from build123d import *

# Parameters (mm, degrees)
BOSS_EXTRUDE1_DEPTH = 1.5
SKETCH2_W           = 1.5
SKETCH2_H           = 5.2
SKETCH2_W_2         = 21.5
SKETCH2_H_2         = 1.5
BOSS_EXTRUDE2_DEPTH = 15


with BuildPart() as part:
    # Sketch1 → Boss-Extrude1 (new body)
    with BuildSketch(Plane.XY):
        Polygon((0, 0), (81.5, 0), (81.5, 13), (79, 13), (79, 10), (76.5, 10), (76.5, 5), (5, 5), (5, 10), (2.5, 10), (2.5, 20.5), (5, 20.5), (5, 25.5), (76.5, 25.5), (76.5, 20.5), (79, 20.5), (79, 17.5), (81.5, 17.5), (81.5, 30.5), (0, 30.5), align=None)
    extrude(amount=BOSS_EXTRUDE1_DEPTH)

    # Sketch2 → Boss-Extrude2 (add)
    with BuildSketch(Plane.XY.offset(1.5)):
        with Locations((0.75, 24.2)):
            Rectangle(SKETCH2_W, SKETCH2_H)
        with Locations((40.75, 0.75)):
            Rectangle(SKETCH2_W_2, SKETCH2_H_2)
        with Locations((80.75, 6.3)):
            Rectangle(SKETCH2_W, SKETCH2_H)
        with Locations((40.75, 29.75)):
            Rectangle(SKETCH2_W_2, SKETCH2_H_2)
        with Locations((80.75, 24.2)):
            Rectangle(SKETCH2_W, SKETCH2_H)
        with Locations((0.75, 6.3)):
            Rectangle(SKETCH2_W, SKETCH2_H)
    extrude(amount=BOSS_EXTRUDE2_DEPTH)


solid = part.part
Design review of the part built by this model. Coordinates are the model's own, in mm. A direction names the side the tool comes from. Round coordinates to 2 decimals unless told otherwise and drop trailing zeros. Order: outer loops, then holes, each group sorted by start corner. A loop starts at its lowest first (then second) coordinate and runs counter-clockwise, first axis right, second up.
1) Consider section C-C (z = 11). State the section outline as (x, y) points.
The answers:
outline: (0, 3.7) - (1.5, 3.7) - (1.5, 8.9) - (0, 8.9) - close; (0, 21.6) - (1.5, 21.6) - (1.5, 26.8) - (0, 26.8) - close; (30, 0) - (51.5, 0) - (51.5, 1.5) - (30, 1.5) - close; (30, 29) - (51.5, 29) - (51.5, 30.5) - (30, 30.5) - close; (80, 3.7) - (81.5, 3.7) - (81.5, 8.9) - (80, 8.9) - close; (80, 21.6) - (81.5, 21.6) - (81.5, 26.8) - (80, 26.8) - close
2) Clearance check with flat-ended pins moving along their axes: pin 1 Ø1.5 at (x, y) = (51.5, 25) entering from +Z; pin 2 Ø1.2 at (x, z) = (80.5, 7.5) entering from +Y; pin 3 Ø1.6 at (y, z) = (29.5, 11.5) entering from +X. State where each tip first meets the part, or that it passes through.
The answers:
pin 1: stops at z = 1.5
pin 2: stops at y = 26.8
pin 3: stops at x = 51.5
3) Consider section B-B (x = 52.5). State the section outline as (y, z) points, plus the area to 3 significant figures.
The answers:
outline: (0, 0) - (5, 0) - (5, 1.5) - (0, 1.5) - close; (25.5, 0) - (30.5, 0) - (30.5, 1.5) - (25.5, 1.5) - close
area: 15.0 mm2
4) Consider section D-D (y = 23). State the section outline as (x, z) points, plus the area to 3 significant figures.
The answers:
outline: (0, 0) - (5, 0) - (5, 1.5) - (1.5, 1.5) - (1.5, 16.5) - (0, 16.5) - close; (76.5, 0) - (81.5, 0) - (81.5, 16.5) - (80, 16.5) - (80, 1.5) - (76.5, 1.5) - close
area: 60.0 mm2
5) Machinability: for faces 1 (the flat face through (80, 24, 9)), 2 (the flat face through (51.5, 1, 9)), 3 (the flat face through (40, 25.5, 1)), 4 (the flat face through (80, 17.5, 1)), 5 (the flat face through (41, 1.5, 9)), which of the approach directions +Z, -Z, +X, -X, +Y, -Y give a long, thin tool a straight path to every point of the face, cutting with its end or side? Answer none if there is none.
The answers:
face 1: +Z, +Y, -Y
face 2: +Z, +X, +Y, -Y
face 3: +Z, -Z
face 4: +Z, -Z, +X
face 5: +Z, +X, -X
6) For L1, parallel to Y at x = 42, z = 8.75; L2, parallel to X at y = 22, z = 3.75; L3, parallel to Z at x = 60, y = 2, list the stretches that pass through material, from the lowest coordinate up.
The answers:
L1: y = 0 to 1.5, 29 to 30.5
L2: x = 0 to 1.5, 80 to 81.5
L3: z = 0 to 1.5
7) Consider section A-A (y = 18.5). State the section outline as (x, z) points, plus the area to 3 significant figures.
The answers:
outline: (0, 0) - (2.5, 0) - (2.5, 1.5) - (0, 1.5) - close; (79, 0) - (81.5, 0) - (81.5, 1.5) - (79, 1.5) - close
area: 7.50 mm2
